```python
from build123d import *

# Parameters (mm, degrees)
F4_DEPTH = 9.652
F5_R     = 4.318
F6_DEPTH = 12.7
F7_R     = 3.048


with BuildPart() as f1:
    # F0 (on Front) → F1 (revolve)
    with BuildSketch(Plane.XZ):
        Polygon((-57.15, -3.048), (-57.15, -15.748), (-15.875, -15.748), (-15.875, 0), (-12.7, 0), (-12.7, 35.052), (-41.275, 35.052), (-41.275, 25.4), (-22.225, 25.4), (-22.225, -3.048), align=None)
    revolve(axis=Axis((0, 0, 1.128893124), (0, 0, -1)))

    # F2 (on face) → F4 (cut, through all)
    with BuildSketch(Plane.XY.offset(35.052)):
        with BuildLine():
            ThreePointArc((-4.7502886947, 32.9331722328), (0, 28.5115), (4.7502886947, 32.9331722328))
            ThreePointArc((4.7502886947, 32.9331722328), (0, 33.274), (-4.7502886947, 32.9331722328))
        make_face()
        with BuildLine():
            ThreePointArc((-4.7502886947, 32.9331722328), (0, 33.274), (4.7502886947, 32.9331722328))
            ThreePointArc((4.7502886947, 32.9331722328), (4.7594461946, 33.1034767737), (4.7625, 33.274))
            ThreePointArc((4.7625, 33.274), (-0.1705232263, 38.0334461946), (-4.7502886947, 32.9331722328))
        make_face()
        with BuildLine():
            ThreePointArc((32.9331722328, -4.7502886947), (33.1886836804, -2.38125), (33.274, 0))
            ThreePointArc((33.274, 0), (33.1886836804, 2.38125), (32.9331722328, 4.7502886947))
            ThreePointArc((32.9331722328, 4.7502886947), (28.5115, 0), (32.9331722328, -4.7502886947))
        make_face()
        with BuildLine():
            ThreePointArc((32.9331722328, 4.7502886947), (33.1886836804, 2.38125), (33.274, 0))
            ThreePointArc((33.274, 0), (33.1886836804, -2.38125), (32.9331722328, -4.7502886947))
            ThreePointArc((32.9331722328, -4.7502886947), (36.5188585492, -3.4860148086), (38.0365, 0))
            ThreePointArc((38.0365, 0), (36.5188585492, 3.4860148086), (32.9331722328, 4.7502886947))
        make_face()
        with BuildLine():
            ThreePointArc((4.7625, -33.274), (4.7594461946, -33.1034767737), (4.7502886947, -32.9331722328))
            ThreePointArc((4.7502886947, -32.9331722328), (0, -33.274), (-4.7502886947, -32.9331722328))
            ThreePointArc((-4.7502886947, -32.9331722328), (-0.1705232263, -38.0334461946), (4.7625, -33.274))
        make_face()
        with BuildLine():
            ThreePointArc((-4.7502886947, -32.9331722328), (0, -33.274), (4.7502886947, -32.9331722328))
            ThreePointArc((4.7502886947, -32.9331722328), (0, -28.5115), (-4.7502886947, -32.9331722328))
        make_face()
        with BuildLine():
            ThreePointArc((-28.5115, 0), (-29.7879851914, 3.2448585492), (-32.9331722328, 4.7502886947))
            ThreePointArc((-32.9331722328, 4.7502886947), (-33.274, 0), (-32.9331722328, -4.7502886947))
            ThreePointArc((-32.9331722328, -4.7502886947), (-29.7879851914, -3.2448585492), (-28.5115, 0))
        make_face()
        with BuildLine():
            ThreePointArc((-32.9331722328, -4.7502886947), (-33.274, 0), (-32.9331722328, 4.7502886947))
            ThreePointArc((-32.9331722328, 4.7502886947), (-38.0365, 0), (-32.9331722328, -4.7502886947))
        make_face()
    extrude(amount=-F4_DEPTH, mode=Mode.SUBTRACT)

    # F5 (on face) → F6 (cut, through all)
    with BuildSketch(Plane.XY.offset(-3.048)):
        with Locations((-23.8125, 41.2444598552)):
            Circle(F5_R)
        with Locations((-47.093068099, 7.0981379266)):
            Circle(F5_R)
        with Locations((-34.9115953959, -32.3932266363)):
            Circle(F5_R)
        with Locations((3.5590207071, -47.4918308408)):
            Circle(F5_R)
        with Locations((39.3496216268, -26.8281177653)):
            Circle(F5_R)
        with Locations((45.5091548756, 14.0377151813)):
            Circle(F5_R)
        with Locations((17.3993662854, 44.3328622792)):
            Circle(F5_R)
    extrude(amount=-F6_DEPTH, mode=Mode.SUBTRACT)

    # F7
    f7_edges = [f1.edges().sort_by_distance(p)[0] for p in [
        (22.225, 0, -3.048),
        (22.225, 0, 25.4),
    ]]
    fillet(f7_edges, radius=F7_R)


solid = f1.part
```
Model file for the job. Use its own axes, mm. A direction names the side the tool comes from. Round coordinates to 2 decimals unless told otherwise and drop trailing zeros. Write each loop counter-clockwise with the first axis right and the second up, starting at its lowest first coordinate (ties: lowest second). Pieces come first, ordered by that corner, then holes. Notation, with made-up numbers: (6.5, -34.5) - (36.5, -34.5) arc R21 ccw to (36.5, -19.5) - close; hole circle Ø3 at (67, -21.5). An arc over 180 degrees is marked (long way). Use CSV: the item, a comma, the result in double quotes. Start each with the question number.
Item 1: Tool access for faces 1 (the face through (3.441, -15.497, -7.764)), 2 (the face through (8.948, -40.293, 30.158)), 3 (the face through (19, -18, 25.4)): list every direction of +Z, -Z, +X, -X, +Y, -Y with a clear straight run to the whole face (end or side of a thin tool).
Item 2: Band-saw the part on A-A (x = 45.5). Write the cut outline in (y, z).
Item 3: Band-saw the part on C-C (z = 2). Write the cut outline in (x, y) (3 decimals), and give its area (3 significant figures).
Item 4: Band-saw the part on B-B (z = -10.5). State how many separate pieces and enclosed holes the cut face has, and give its area (3 significant figures).
Item 5: Pin check, flat tips, straight feed: P1, Ø5, axis at x = 3, z = 14.5, coming from the -Y side; P2, Ø1, axis at x = -13.5, z = 29.5, coming from the +Y side; P3, Ø5, axis at x = 15, z = -5, coming from the -Y side. Stop position of each tip, or through.
Item 6: Two-plate mould, pull along Z, no slides. Class faces 4 (the face through (-51.407, 7.288, -9.309)), 5 (the face through (-10, -9, 35.052)), 6 (the face through (12, -25, -3.048)), 7 (the face through (-21.199, 6.676, 11.02)): released by +Z, released by -Z, zero draft, split by the parting line, or undercut.
Item 7: Drill centre lines: L1, parallel to Z at x = -26, y = 7.5; L2, parallel to Z at x = 43.5, y = -1.5; L3, parallel to X at y = -4, z = 33. Where is each one in solid material? Low to high. Write a range as [from, to].
Checked values:
1,face 1,"-Z"
1,face 2,"+Z"
1,face 3,"none"
2,outline,"(-34.58, -15.75) - (9.72, -15.75) - (9.72, -3.05) - (-34.58, -3.05) - close; (18.36, -15.75) - (34.58, -15.75) - (34.58, -3.05) - (18.36, -3.05) - close"
3,outline,"circle Ø44.45 at (0, 0); hole circle Ø25.4 at (0, 0)"
3,area,"1,050 mm²"
4,separate pieces,"1"
4,enclosed holes,"8"
4,area,"9,060 mm²"
5,P1,"stops at y = -22.22"
5,P2,"stops at y = 39.17"
5,P3,"stops at y = -55.77"
6,face 4,"zero draft"
6,face 5,"released by +Z"
6,face 6,"undercut"
6,face 7,"undercut"
7,L1,"z = [-15.75, -3.05], [25.4, 35.05]"
7,L2,"z = [-15.75, -3.05]"
7,L3,"x = [-41.08, -35.86], [-30.69, -12.05], [12.05, 30.69], [35.86, 41.08]"
